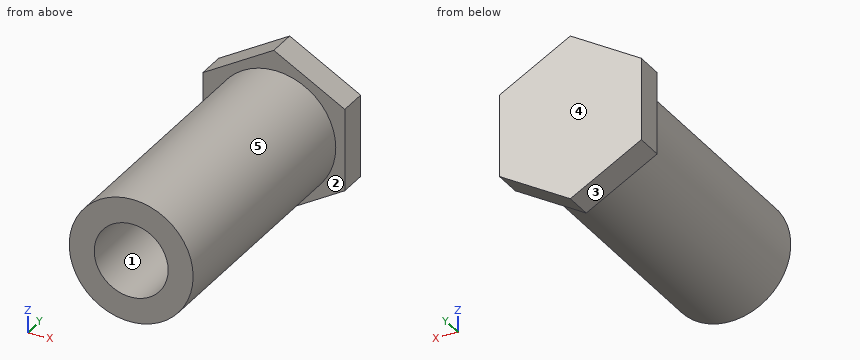
from build123d import *

# Parameters (mm, degrees)
CROQUIS1_W                = 2.095
CROQUIS1_H                = 10
SALIENTE_EXTRUIR1_DEPTH   = 1
TALADRO_ROSCADO_M31_D     = 2.5
TALADRO_ROSCADO_M31_DEPTH = 4
TALADRO_ROSCADO_M31_TIP   = 0.751075774


with BuildPart() as part:
    # Croquis1 → Revolución1 (revolve)
    with BuildSketch(Plane.XY):
        with Locations((1.0475, -5)):
            Rectangle(CROQUIS1_W, CROQUIS1_H)
    revolve(axis=Axis((0, 0, 0), (0, -1, 0)))

    # Croquis2 → Saliente-Extruir1 (add)
    with BuildSketch(Plane(origin=(0, 0, 0), x_dir=(1, 0, 0), z_dir=(0, 1, 0))):
        Polygon((2.4, -1.385640646), (2.4, 1.385640646), (0, 2.771281292), (-2.4, 1.385640646), (-2.4, -1.385640646), (0, -2.771281292), align=None)
    extrude(amount=-SALIENTE_EXTRUIR1_DEPTH)

    # Taladro roscado M31
    with Locations(Plane(origin=(0, -10, 0), x_dir=(-1, 0, 0), z_dir=(0, -1, 0))):
        with Locations((0, 0)):
            Hole(TALADRO_ROSCADO_M31_D / 2, depth=TALADRO_ROSCADO_M31_DEPTH)
            with Locations((0, 0, -(TALADRO_ROSCADO_M31_DEPTH + TALADRO_ROSCADO_M31_TIP / 2))):  # 118° drill point
                Cone(0, TALADRO_ROSCADO_M31_D / 2, TALADRO_ROSCADO_M31_TIP, mode=Mode.SUBTRACT)


solid = part.part
For this review, take the finished solid that the model builds, in its own axes (mm). Face numbers are marked on the shaded views. A direction names the side the tool comes from. Round coordinates to 2 decimals unless told otherwise and drop trailing zeros. Loops run counter-clockwise (first coordinate to the right, second up) from the corner with the lowest first, then second, coordinate; pieces in that order, holes last. Notation, with made-up numbers: (-6.5, 76.25) - (9.5, 76.25) arc R17 ccw to (9.5, 91.25) - close; hole circle Ø5 at (77.25, -21). An arc over 180 degrees is marked (long way). Answer as CSV lines item,"result".
(1) Insertion check: P1, Ø1.5, axis at x = 0.5, y = -5, coming from the +Z side (3 decimals). The pin has a flat end and moves straight along its axis. Give the tip position at first contact, or say it passes through.
Checked values:
P1,"stops at z = 2.095"
(2) Wall thickness on line 1 (Z direction, x = 0, y = -7.4) (3 decimals); line 2 (Y direction, x = -0.3, z = 2.55); line 3 (X direction, y = -8.25, z = 1): over which ranges is each line inside the solid? List them lowest first.
Checked values:
line 1,"z = -2.095 to -1.25, 1.25 to 2.095"
line 2,"y = -1 to 0"
line 3,"x = -1.84 to -0.75, 0.75 to 1.84"
(3) Tool access review of the marked faces 4 and 5: name each direction out of +Z, -Z, +X, -X, +Y, -Y from which nothing blocks a thin tool from reaching the whole face with its end or side.
Checked values:
face 4,"+Z, -Z, +X, -X, +Y"
face 5,"-Y"
(4) Consider section B-B on z = -1.7. Give the boundary of the cut face in (x, y).
Checked values:
outline,"(-1.86, -1) - (-1.22, -1) - (-1.22, -10) - (1.22, -10) - (1.22, -1) - (1.86, -1) - (1.86, 0) - (-1.86, 0) - close"
(5) Consider section D-D on y = -5.5. Give the boundary of the cut face in (x, z) (3 decimals).
Checked values:
outline,"circle Ø4.19 at (0, 0); hole circle Ø0.836 at (0, 0)"
(6) Mouldability with a two-part tool opening along Z and no side actions: class the marked faces 1, 2 and 3 as +Z half, -Z half, draft (parallel to the pull), parting line (faces both ways), or undercut.
Checked values:
face 1,"undercut"
face 2,"draft"
face 3,"-Z half"
(7) Consider section C-C on y = -3.5. Give the boundary of the cut face in (x, z) (3 decimals).
Checked values:
outline,"circle Ø4.19 at (0, 0)"
(8) Consider section A-A on x = 1.75. Give the boundary of the cut face in (y, z).
Checked values:
outline,"(-10, -1.15) - (-1, -1.15) - (-1, -1.76) - (0, -1.76) - (0, 1.76) - (-1, 1.76) - (-1, 1.15) - (-10, 1.15) - close"
